Autodesk Inventor part; units mm, degrees
ref_plane "YZ Plane" through (0, 0, 0) normal (1, 0, 0) x (0, 1, 0)
ref_plane "XZ Plane" through (0, 0, 0) normal (0, 1, 0) x (-1, 0, 0)
ref_plane "XY Plane" through (0, 0, 0) normal (0, 0, 1) x (1, 0, 0)
sketch "Sketch2" plane through (0, 0, 0) normal (0, 1, 0) x (-1, 0, 0)
  line L0 (15, 20.15) -> (20.15, 15)
  line L1 (20.15, 15) -> (20.15, -15)
  line L2 (20.15, -15) -> (15, -20.15)
  line L3 (15, -20.15) -> (-15, -20.15)
  line L4 (-15, -20.15) -> (-20.15, -15)
  line L5 (-20.15, -15) -> (-20.15, 15)
  line L6 (-20.15, 15) -> (-15, 20.15)
  line L7 (-15, 20.15) -> (15, 20.15)
  point P0 (0, 0)
  point P1 (20.15, 0)
  point P2 (0, -20.15)
  dimension "d2" = 30
  dimension "d3" = 40.3
  dimension "d4" = 135
extrude "Extrusion1" add sketch "Sketch2" along normal mid plane 34
sketch "Sketch7" plane through (0, 17, 0) normal (0, 1, 0) x (1, 0, 0)
  circle A0 centre (0, 0) radius 11
  dimension "d27" = 22
extrude "Extrusion3" add sketch "Sketch7" along normal blind 2
sketch "Sketch8" plane through (0, 19, 0) normal (0, 1, 0) x (1, 0, 0)
  circle A0 centre (0, 0) radius 4
  dimension "d30" = 8
extrude "Extrusion4" cut sketch "Sketch8" against normal blind 1
sketch "Sketch9" plane through (0, 18, 0) normal (0, 1, 0) x (1, 0, 0)
  circle A0 centre (0, 0) radius 2.5
  dimension "d33" = 5
extrude "Extrusion5" add sketch "Sketch9" along normal blind 22
sketch "Sketch10" plane through (-15, 17, 20.15) normal (0, 0, 1) x (1, 0, 0)
  line L0 (30, 0) -> (30, -34)
  line L1 (0, 0) -> (30, 0)
  line L2 (0, -34) -> (0, 0)
  line L3 (30, -34) -> (0, -34)
  line L4 (0, 0) -> (30, 0)
  line L5 (30, 0) -> (30, -10)
  line L6 (30, -10) -> (0, -10)
  line L7 (0, -10) -> (0, 0)
  line L8 (0, 0) -> (30, -10) construction
  line L9 (30, 0) -> (0, -10) construction
  line L10 (0, -24) -> (30, -24)
  line L11 (30, -24) -> (30, -34)
  line L12 (30, -34) -> (0, -34)
  line L13 (0, -34) -> (0, -24)
  line L14 (0, -24) -> (30, -34) construction
  line L15 (30, -24) -> (0, -34) construction
  line L16 (0, 0) -> (30, 0)
  point P0 (15, -17)
  point P1 (15, -5)
  point P2 (15, -29)
  dimension "d36" = 10
  dimension "d37" = 10
extrude "Extrusion6" add sketch "Sketch10" along normal blind 1 contours L0 L6 L2 L1 | L0 L3 L2 L10
mirror "Mirror1" about plane through (0, 0, 0) normal (0, 0, 1) of "Extrusion6"
sketch "Sketch11" plane through (20.15, -17, -15) normal (1, 0, 0) x (0, 0, -1)
  line L0 (0, 34) -> (0, 0)
  line L1 (-30, 34) -> (0, 34)
  line L2 (-30, 34) -> (-30, 0)
  line L3 (0, 0) -> (-30, 0)
  line L4 (-30, 34) -> (0, 34)
  line L5 (0, 34) -> (0, 24)
  line L6 (0, 24) -> (-30, 24)
  line L7 (-30, 24) -> (-30, 34)
  line L8 (-30, 34) -> (0, 24) construction
  line L9 (0, 34) -> (-30, 24) construction
  line L10 (-30, 10) -> (0, 10)
  line L11 (0, 10) -> (0, 0)
  line L12 (0, 0) -> (-30, 0)
  line L13 (-30, 0) -> (-30, 10)
  line L14 (-30, 10) -> (0, 0) construction
  line L15 (0, 10) -> (-30, 0) construction
  line L16 (-30, 34) -> (0, 34)
  point P0 (-15, 17)
  point P1 (-15, 29)
  point P2 (-15, 5)
  dimension "d40" = 10
extrude "Extrusion7" add sketch "Sketch11" along normal blind 1 contours L0 L6 L2 L1 | L0 L3 L2 L10
mirror "Mirror2" about plane through (0, 0, 0) normal (1, 0, 0) of "Extrusion7"
sketch "Sketch12" plane through (-15, -7, 20.15) normal (-0.7071, 0, 0.7071) x (0.7071, 0, 0.7071)
  line L0 (0, -10) -> (0, 0)
  line L1 (0, 0) -> (0, 14)
  line L2 (0, 14) -> (0, 24)
  line L3 (-7.2832, 24) -> (0, 24)
  line L4 (-7.2832, 24) -> (-7.2832, 14)
  line L5 (-7.2832, 14) -> (-7.2832, 0)
  line L6 (-7.2832, 0) -> (-7.2832, -10)
  line L7 (0, -10) -> (-7.2832, -10)
  line L8 (-7.2832, 24) -> (0, 24)
  line L9 (0, 24) -> (0, 14)
  line L10 (0, 14) -> (-7.2832, 14)
  line L11 (-7.2832, 14) -> (-7.2832, 24)
  line L12 (-7.2832, 24) -> (0, 14) construction
  line L13 (0, 24) -> (-7.2832, 14) construction
  line L14 (-7.2832, 0) -> (0, 0)
  line L15 (0, 0) -> (0, -10)
  line L16 (0, -10) -> (-7.2832, -10)
  line L17 (-7.2832, -10) -> (-7.2832, 0)
  line L18 (-7.2832, 0) -> (0, -10) construction
  line L19 (0, 0) -> (-7.2832, -10) construction
  line L20 (-7.2832, 24) -> (0, 24)
  line L21 (0, -10) -> (-7.2832, -10)
  point P0 (-3.6416, 7)
  point P1 (-3.6416, 19)
  point P2 (-3.6416, -5)
  dimension "d43" = 10
  dimension "d44" = 10
extrude "Extrusion8" add sketch "Sketch12" along normal blind 1 contours L7 L6 L14 L0 | L10 L4 L3 L2
sketch "Sketch14" plane through (-15, 7, 21.15) normal (-1, 0, 0) x (0, 0, 1)
  line L0 (-1, 0) -> (-1, 10)
  line L1 (-1, 0) -> (0, 0)
  line L2 (0, 10) -> (0, 0)
  line L3 (-1, 10) -> (0, 10)
  line L4 (-1, -24) -> (-1, -14)
  line L5 (-1, -24) -> (0, -24)
  line L6 (0, -14) -> (0, -24)
  line L7 (-1, -14) -> (0, -14)
  point P0 (-21.15, -7)
extrude "Extrusion9" add sketch "Sketch14" along normal up to surface surface through (-18.2821, 12, 18.2821) normal (-0.7071, 0, 0.7071)
sketch "Sketch15" plane through (-21.15, 7, 15) normal (0, 0, 1) x (1, 0, 0)
  line L0 (1, 10) -> (1, 0)
  line L1 (1, 10) -> (0, 10)
  line L2 (0, 10) -> (0, 0)
  line L3 (1, 0) -> (0, 0)
  line L4 (1, -14) -> (1, -24)
  line L5 (1, -14) -> (0, -14)
  line L6 (0, -14) -> (0, -24)
  line L7 (1, -24) -> (0, -24)
  point P0 (21.15, -7)
extrude "Extrusion10" add sketch "Sketch15" along normal up to surface surface through (-18.2821, -12, 18.2821) normal (-0.7071, 0, 0.7071)
mirror "Mirror3" about plane through (0, 0, 0) normal (1, 0, 0) of "Extrusion8", "Extrusion9", "Extrusion10"
mirror "Mirror4" about plane through (0, 0, 0) normal (0, 0, 1) of "Extrusion8", "Extrusion9", "Extrusion10", "Mirror3"
sketch "Sketch17" plane through (0, 17, 0) normal (0, 1, 0) x (1, 0, 0)
  line L0 (-21.15, -15.4142) -> (-15.4142, -21.15)
  line L1 (-15.4142, -21.15) -> (15.4142, -21.15)
  line L2 (21.15, -15.4142) -> (15.4142, -21.15)
  line L3 (21.15, -15.4142) -> (21.15, 15.4142)
  line L4 (21.15, 15.4142) -> (15.4142, 21.15)
  line L5 (15.4142, 21.15) -> (-15.4142, 21.15)
  line L6 (-21.15, 15.4142) -> (-15.4142, 21.15)
  line L7 (-21.15, 15.4142) -> (-21.15, -15.4142)
  circle A0 centre (0, 0) radius 11
  circle A1 centre (-15.5, -15.5) radius 1.5
  circle A2 centre (-15.5, 15.5) radius 1.5
  circle A3 centre (15.5, 15.5) radius 1.5
  circle A4 centre (15.5, -15.5) radius 1.5
  dimension "d53" = 3
  dimension "d54" = 31
  dimension "d55" = 31
  dimension "d57" = 15.5
  dimension "d66" = 15.5
hole "Hole3" at (-15.5, 17, 15.5) at (-15.5, 17, -15.5) at (15.5, 17, -15.5) at (15.5, 17, 15.5) direction (0, -1, 0) diameter 3 depth 4.5
ref_plane "Work Plane4" through (0, 18, 0) normal (1, 0, 0) x (0, 1, 0)
ref_plane "Work Plane1" through (0, 0, 0) normal (1, 0, 0) x (0, 1, 0)
ref_plane "Work Plane2" through (0, 0, 0) normal (-1, 0, 0) x (0, 1, 0)
ref_plane "Work Plane3" through (0, 0, 0) normal (-1, 0, 0) x (0, 1, 0)
properties part number "Motor_paso"
Model file for the job. Use its own axes, mm. A direction names the side the tool comes from. Coordinates: 2 decimals unless noted, no trailing zeros. Order: outer loops, then holes, each group sorted by start corner. A loop starts at its lowest first (then second) coordinate and runs counter-clockwise, first axis right, second up. Notation, with made-up numbers: (83.5, 38) - (100.5, 38) arc R17 cw to (100.5, 65) - close; hole circle Ø2 at (3, 79.25). An arc over 180 degrees is marked (long way). Return JSON: item names as keys, results as strings. Group by question number.
1) Flat gauge pins, fed straight in: P1, Ø24, axis at x = -4, z = -2.5, coming from the +Y side; P2, Ø2.5, axis at x = 15.5, z = -15.5, coming from the +Y side; P3, Ø4, axis at x = 3.5, z = 17, coming from the +Y side; P4, Ø7, axis at x = -0.5, y = 0, coming from the -Z side. Where does each tip first touch, or does it go through?
2) Tool access for faces 1 (the cylindrical face through (15.43, 14.72, 14)), 2 (the flat face through (-17.54, -0.1, 17.61)), 3 (the flat face through (-18.322, -11.93, 18.242)): list every direction of +Z, -Z, +X, -X, +Y, -Y with a clear straight run to the whole face (end or side of a thin tool).
3) Saw through at C-C, the plane z = 0. Write the cut outline in (x, y), plus the area to 3 significant figures.
4) Saw through at A-A, the plane x = 13. Write the cut outline in (y, z), plus the area to 3 significant figures.
5) Saw through at D-D, the plane x = 0. Write the cut outline in (y, z).
6) Saw through at B-B, the plane y = 6. Write the cut outline in (x, z).
7) Mould opens along Y. For faces 4 (the flat face through (-16, 12.5, -16)), 5 (the flat face through (0, -12, 21.15)), 6 (the flat face through (17.54, -0.1, -17.61)) say: released by +Y, released by -Y, zero draft, split by the parting line, or undercut.
8) Probe line 1 (Z direction, x = 0, y = 18.4); line 2 (X direction, y = 15.45, z = 15.5). List the from-to ranges inside material, lowest first. Write a range as from..to.
Values found:
{
 "1": {"P1": "stops at y = 40", "P2": "stops at y = 12.5", "P3": "stops at y = 17", "P4": "stops at z = -20.15"},
 "2": {"face 1": "+Y", "face 2": "+Z, -X", "face 3": "+Z, -X, +Y, -Y"},
 "3": {"outline": "(-21.15, -17) - (21.15, -17) - (21.15, -7) - (20.15, -7) - (20.15, 7) - (21.15, 7) - (21.15, 17) - (11, 17) - (11, 19) - (4, 19) - (4, 18) - (2.5, 18) - (2.5, 40) - (-2.5, 40) - (-2.5, 18) - (-4, 18) - (-4, 19) - (-11, 19) - (-11, 17) - (-21.15, 17) - (-21.15, 7) - (-20.15, 7) - (-20.15, -7) - (-21.15, -7) - close", "area": "1,560 mm²"},
 "4": {"outline": "(-17, -21.15) - (-7, -21.15) - (-7, -20.15) - (7, -20.15) - (7, -21.15) - (17, -21.15) - (17, 21.15) - (7, 21.15) - (7, 20.15) - (-7, 20.15) - (-7, 21.15) - (-17, 21.15) - close", "area": "1,410 mm²"},
 "5": {"outline": "(-17, -21.15) - (-7, -21.15) - (-7, -20.15) - (7, -20.15) - (7, -21.15) - (17, -21.15) - (17, -11) - (19, -11) - (19, -4) - (18, -4) - (18, -2.5) - (40, -2.5) - (40, 2.5) - (18, 2.5) - (18, 4) - (19, 4) - (19, 11) - (17, 11) - (17, 21.15) - (7, 21.15) - (7, 20.15) - (-7, 20.15) - (-7, 21.15) - (-17, 21.15) - close"},
 "6": {"outline": "(-20.15, -15) - (-15, -20.15) - (15, -20.15) - (20.15, -15) - (20.15, 15) - (15, 20.15) - (-15, 20.15) - (-20.15, 15) - close"},
 "7": {"face 4": "released by +Y", "face 5": "zero draft", "face 6": "undercut"},
 "8": {"line 1": "z = -11..-4, -2.5..2.5, 4..11", "line 2": "x = -21.06..-17, -14..14, 17..21.06"}
}
